from build123d import *

# Parameters (mm, degrees)
SKETCH1_W      = 22.86
SKETCH1_H      = 20.32
EXTRUDE1_DEPTH = 1.7
SKETCH2_W      = 2.6
SKETCH2_H      = 20.32
EXTRUDE2_DEPTH = 8.4


with BuildPart() as part:
    # Sketch1 → Extrude1 (new body)
    with BuildSketch(Plane(origin=(0, 0, 0), x_dir=(1, 0, 0), z_dir=(0, 1, 0))):
        with Locations((-18.208858156, -4.831082697)):
            Rectangle(SKETCH1_W, SKETCH1_H)
    extrude(amount=EXTRUDE1_DEPTH)

    # Sketch2 → Extrude2 (add)
    with BuildSketch(Plane.XZ):
        with Locations((-28.338858156, 4.831082697)):
            Rectangle(SKETCH2_W, SKETCH2_H)
    extrude(amount=EXTRUDE2_DEPTH)


solid = part.part
Geometry: final body of the model. Coordinates: model frame, mm. A direction names the side the tool comes from. Coordinates: 2 decimals unless noted, no trailing zeros. Loops run counter-clockwise (first coordinate to the right, second up) from the corner with the lowest first, then second, coordinate; pieces in that order, holes last. Notation, with made-up numbers: (63, 85) - (84, 85) arc R28 ccw to (84, 122) - close; hole circle Ø7 at (48.25, 24.5). An arc over 180 degrees is marked (long way). One line per question, with ' | ' between items. Start each with the question number.
(1) Reachability of faces 1 (the flat face through (-17, 0, 5)), 2 (the flat face through (-28, -8.4, 5)) from +Z, -Z, +X, -X, +Y, -Y: full face, straight path, thin tool, end or side. Return the list, or none.
(2) First-contact query: pin 1 (5 mm diameter, centred on y = -4, z = 8.5, fed in from +X). Flat tip, straight axial feed; report the tip coordinate or a pass-through.
(3) Cut plane C-C on y = -2.5. Output: boundary loops of the cut face in (x, z).
(4) Ray query, L1, parallel to X at y = -1.5, z = 2.5; L2, parallel to Y at x = -16.25, z = 10.75. Return the intervals inside material, ascending. Write a range as from..to.
(5) Cut plane B-B on x = -20.5. Output: boundary loops of the cut face in (y, z).
(6) Cut plane A-A on z = -2.5. Output: boundary loops of the cut face in (x, y).
Here are the results:
1) face 1: +Z, -Z, +X, -Y | face 2: +Z, -Z, +X, -X, -Y
2) pin 1: x = -27.04
3) outline: (-29.64, -5.33) - (-27.04, -5.33) - (-27.04, 14.99) - (-29.64, 14.99) - close
4) L1: -29.64..-27.04 | L2: 0..1.7
5) outline: (0, -5.33) - (1.7, -5.33) - (1.7, 14.99) - (0, 14.99) - close
6) outline: (-29.64, -8.4) - (-27.04, -8.4) - (-27.04, 0) - (-6.78, 0) - (-6.78, 1.7) - (-29.64, 1.7) - close
